```python
from build123d import *

# Parameters (mm, degrees)
SKETCH_1_R          = 3.2
EXTRUDE_1_DEPTH     = 10
SKETCH_2_R          = 5.25
CUT_EXTRUDE_1_DEPTH = 7
SKETCH_3_R          = 3.25
CUT_EXTRUDE_2_DEPTH = 10
SKETCH_4_R          = 3.25
SKETCH_4_W          = 10.4
SKETCH_4_H          = 10.4
CUT_EXTRUDE_3_DEPTH = 7
EXTRUDE_2_DEPTH     = 10


with BuildPart() as part:
    # 스케치1 → 보스-돌출1 (new body)
    with BuildSketch(Plane(origin=(0, 0, 0), x_dir=(1, 0, 0), z_dir=(0, 1, 0))):
        with BuildLine():
            Line((-7.071067812, 7.071067812), (-67.705474299, -53.563338675))
            ThreePointArc((-67.705474299, -53.563338675), (-70.634406487, -60.634406487), (-67.705474299, -67.705474299))
            ThreePointArc((-67.705474299, -67.705474299), (0, -95.75), (67.705474299, -67.705474299))
            ThreePointArc((67.705474299, -67.705474299), (70.634406487, -60.634406487), (67.705474299, -53.563338675))
            Line((67.705474299, -53.563338675), (7.071067812, 7.071067812))
            ThreePointArc((7.071067812, 7.071067812), (0, 10), (-7.071067812, 7.071067812))
        make_face()
        with Locations((-8.75, -58.75)):
            Circle(SKETCH_1_R, mode=Mode.SUBTRACT)
        with Locations((-8.75, -8.75)):
            Circle(SKETCH_1_R, mode=Mode.SUBTRACT)
        with Locations((-58.75, -58.75)):
            Circle(SKETCH_1_R, mode=Mode.SUBTRACT)
        with Locations((41.25, -58.75)):
            Circle(SKETCH_1_R, mode=Mode.SUBTRACT)
    extrude(amount=EXTRUDE_1_DEPTH)

    # 스케치2 → 컷-돌출1 (cut)
    with BuildSketch(Plane(origin=(0, 10, 0), x_dir=(1, 0, 0), z_dir=(0, 1, 0))):
        with Locations((-8.75, -8.75)):
            Circle(SKETCH_2_R)
        with Locations((-58.75, -58.75)):
            Circle(SKETCH_2_R)
        with Locations((41.25, -58.75)):
            Circle(SKETCH_2_R)
        with Locations((-8.75, -58.75)):
            Circle(SKETCH_2_R)
    extrude(amount=-CUT_EXTRUDE_1_DEPTH, mode=Mode.SUBTRACT)

    # 스케치3 → 컷-돌출2 (cut)
    with BuildSketch(Plane(origin=(0, 10, 0), x_dir=(1, 0, 0), z_dir=(0, 1, 0))):
        Circle(SKETCH_3_R)
        with Locations((0, -87.5)):
            Circle(SKETCH_3_R)
    extrude(amount=-CUT_EXTRUDE_2_DEPTH, mode=Mode.SUBTRACT)

    # 스케치4 → 컷-돌출3 (cut)
    with BuildSketch(Plane.XZ):
        Polygon((0, 7.353910524), (-7.353910524, 0), (0, -7.353910524), (7.353910524, 0), align=None)
        Circle(SKETCH_4_R, mode=Mode.SUBTRACT)
        with Locations((0, 87.5)):
            Rectangle(SKETCH_4_W, SKETCH_4_H)
        with Locations((0, 87.5)):
            Circle(SKETCH_4_R, mode=Mode.SUBTRACT)
    extrude(amount=-CUT_EXTRUDE_3_DEPTH, mode=Mode.SUBTRACT)

    # 스케치5 → 보스-돌출2 (add)
    with BuildSketch(Plane(origin=(0, 10, 0), x_dir=(1, 0, 0), z_dir=(0, 1, 0))):
        with BuildLine():
            Line((0.505263158, -95.998670351), (0.5, -94.998684201))
            ThreePointArc((0.5, -94.998684201), (0, -95), (-0.5, -94.998684201))
            Line((-0.5, -94.998684201), (-0.505263158, -95.998670351))
            ThreePointArc((-0.505263158, -95.998670351), (0, -96), (0.505263158, -95.998670351))
        make_face()
    extrude(amount=-EXTRUDE_2_DEPTH)


solid = part.part
```
Check sheet for the modelled part. Datum: model origin and axes. Units: mm. A direction names the side the tool comes from. Give positions to 0.01 mm unless a question says otherwise; leave off trailing zeros. Write each loop counter-clockwise with the first axis right and the second up, starting at its lowest first coordinate (ties: lowest second). Pieces come first, ordered by that corner, then holes.
Item 1: Cross-section at C-C (z = 87.5). Enter the section's corners in (x, y), and give its area (3 significant figures).
Item 2: Cross-section at B-B (y = 4.75). Enter the section's corners in (x, z), and give its area (3 significant figures).
Item 3: Access from +Z, -Z, +X, -X, +Y, -Y to the whole of each face (thin tool, end or side, straight path). Record for faces 5 (the face through (40.112, 6.549, 63.875)), 6 (the face through (3.625, 3.451, -3.728)), 7 (the face through (37.81, 4.93, 23.67)).
Item 4: Scan lines: L1, parallel to X at y = 8.25, z = 55; L2, parallel to Z at x = -8.75, y = 7.5; L3, parallel to X at y = 1.1, z = 58.75. Record each from-to range of solid material in increasing order.
Item 5: Draft check along X on faces 1 (the face through (-1, 10, 54)), 2 (the face through (-37.36, 4.93, 88.16)), 3 (the face through (0, 5, -10)), 4 (the face through (0, 3, 92.7)). Enter one of: released by +X, released by -X, zero draft, split by the parting line, or undercut.
Item 6: Gauge pin test, flat ends, axial feed: pin 1 (7.5 mm diameter, centred on x = 0, z = 0, fed in from -Y); pin 2 (5 mm diameter, centred on x = -30.5, y = 6.5, fed in from +Z); pin 3 (2 mm diameter, centred on x = -2, y = 3, fed in from -Z). Record the tip position at first contact, or that the pin passes through.
Item 7: Cross-section at D-D (z = 58.75). Enter the section's corners in (x, y), and give its area (3 significant figures).
Item 8: Cross-section at A-A (x = 41.25). Enter the section's corners in (y, z), and give its area (3 significant figures).
Report:
1. outline: (-38.88, 0) - (-5.2, 0) - (-5.2, 7) - (-3.25, 7) - (-3.25, 10) - (-38.88, 10) - close; (3.25, 7) - (5.2, 7) - (5.2, 0) - (38.88, 0) - (38.88, 10) - (3.25, 10) - close
1. area: 685 mm2
2. outline: (-67.71, 53.56) - (-7.07, -7.07) arc R10 ccw to (7.07, -7.07) - (67.71, 53.56) arc R10 ccw to (67.71, 67.71) arc R95.75 ccw to (0.5, 95.75) - (0.51, 96) arc R96 ccw to (-0.51, 96) - (-0.5, 95.75) arc R95.75 ccw to (-67.71, 67.71) arc R10 ccw to start; hole circle Ø10.5 at (-58.75, 58.75); hole circle Ø10.5 at (-8.75, 8.75); hole circle Ø10.5 at (-8.75, 58.75); hole (-7.35, 0) - (0, -7.35) - (7.35, 0) - (0, 7.35) - close; hole (-5.2, 82.3) - (5.2, 82.3) - (5.2, 92.7) - (-5.2, 92.7) - close; hole circle Ø10.5 at (41.25, 58.75)
2. area: 8,590 mm2
3. face 5: +Y
3. face 6: -Y
3. face 7: -Z, +X, +Y, -Y
4. L1: x = -68.9 to -62.42, -55.08 to -12.42, -5.08 to 37.58, 44.92 to 68.9
4. L2: z = -5.39 to 3.5, 14 to 53.5, 64 to 95.35
4. L3: x = -70.46 to -61.95, -55.55 to -11.95, -5.55 to 38.05, 44.45 to 70.46
5. face 1: zero draft
5. face 2: released by -X
5. face 3: split by the parting line
5. face 4: undercut
6. pin 1: stops at y = 7
6. pin 2: stops at z = 91.56
6. pin 3: stops at z = -9.95
7. outline: (-70.46, 0) - (-61.95, 0) - (-61.95, 3) - (-64, 3) - (-64, 10) - (-70.46, 10) - close; (-55.55, 0) - (-11.95, 0) - (-11.95, 3) - (-14, 3) - (-14, 10) - (-53.5, 10) - (-53.5, 3) - (-55.55, 3) - close; (-5.55, 0) - (38.05, 0) - (38.05, 3) - (36, 3) - (36, 10) - (-3.5, 10) - (-3.5, 3) - (-5.55, 3) - close; (44.45, 0) - (70.46, 0) - (70.46, 10) - (46.5, 10) - (46.5, 3) - (44.45, 3) - close
7. area: 1,130 mm2
8. outline: (0, 27.11) - (10, 27.11) - (10, 53.5) - (3, 53.5) - (3, 55.55) - (0, 55.55) - close; (0, 61.95) - (3, 61.95) - (3, 64) - (10, 64) - (10, 86.41) - (0, 86.41) - close
8. area: 500 mm2
